Design review of the part built by this model. Coordinates are the model's own, in mm. Coordinates: 2 decimals unless noted, no trailing zeros. Loops run counter-clockwise (first coordinate to the right, second up) from the corner with the lowest first, then second, coordinate; pieces in that order, holes last. Notation, with made-up numbers: M 28.25,19.5 L 42.25,19.5 A7 ccw 42.25,31.5 Z; hole C 40.5,42.5 d2. An arc over 180 degrees is marked long. Write item = value, one per line. Start each with the question number.
from build123d import *

# Parameters (mm, degrees)
F0_R     = 12.7
F1_DEPTH = 6.35


with BuildPart() as f1:
    # F0 (on Top) → F1 (new body)
    with BuildSketch(Plane.XY):
        Polygon((86.252718, 34.973921), (-60.852718, 34.973921), (-116.947282, -62.184713), (-43.394563, -189.581758), (68.794563, -189.581758), (142.347282, -62.184713), align=None)
        with Locations((12.7, -72.264184)):
            Circle(F0_R, mode=Mode.SUBTRACT)
        Polygon((-116.947282, -62.184713), (-60.852718, 34.973921), (-69.651536, 34.973921), (-121.346691, -54.564713), align=None)
        Polygon((95.051536, 34.973921), (86.252718, 34.973921), (142.347282, -62.184713), (146.746691, -54.564713), align=None)
        Polygon((68.794563, -189.581758), (-43.394563, -189.581758), (-38.995154, -197.201758), (64.395154, -197.201758), align=None)
    extrude(amount=F1_DEPTH)


solid = f1.part
Q1. Add section B-B on z = 4. State the section outline as (x, y) points.
Q2. To check wall thickness, follow line 1 (Y direction, x = 12.7, z = 2.5); line 2 (X direction, y = -64, z = 4.25); line 3 (Y direction, x = -105.5, z = 3.5). State the ranges of each line that lie inside material, in increasing order. Write a range as from..to.
Q3. Clearance check with flat-ended pins moving along their axes: P1, Ø2, axis at x = 86.5, z = 3, coming from the -Y side; P2, Ø1, axis at y = 8.5, z = 3.5, coming from the -X side. State where each tip first meets the part, or that it passes through.
Q4. Add section A-A on x = 12.7. State the section outline as (y, z) points, plus the area to 3 significant figures.
Q5. Add section D-D on x = 110.5. State the section outline as (y, z) points.
Q6. Add section C-C on y = -133. State the section outline as (x, z) points.
Q7. Mouldability with a two-part tool opening along Y and no side actions: class faces 1 (the face through (14, 34.974, 3)), 2 (the face through (11.05, -59.67, 3.13)), 3 (the face through (11, -54, 6.35)) as released by +Y, released by -Y, zero draft, split by the parting line, or undercut.
Values follow:
q1.outline = M -121.35,-54.56 L -39,-197.2 L 64.4,-197.2 L 146.75,-54.56 L 95.05,34.97 L -69.65,34.97 Z; hole C 12.7,-72.26 d25.4
q2.line_1 = -197.2..-84.96, -59.56..34.97
q2.line_2 = -115.9..3.06, 22.34..141.3
q2.line_3 = -82.01..-27.12
q3.P1 = -160.65
q3.P2 = -85.22
q4.outline = M -197.2,0 L -84.96,0 L -84.96,6.35 L -197.2,6.35 Z; M -59.56,0 L 34.97,0 L 34.97,6.35 L -59.56,6.35 Z
q4.area = 1,310 mm2
q5.outline = M -117.35,0 L 8.22,0 L 8.22,6.35 L -117.35,6.35 Z
q6.outline = M -76.06,0 L 101.46,0 L 101.46,6.35 L -76.06,6.35 Z
q7.face_1 = released by +Y
q7.face_2 = undercut
q7.face_3 = zero draft
